Can you work these out from the model? Positions are in its coordinate system, mm. A direction names the side the tool comes from. Coordinates: 2 decimals unless noted, no trailing zeros. Order: outer loops, then holes, each group sorted by start corner. A loop starts at its lowest first (then second) coordinate and runs counter-clockwise, first axis right, second up.
```python
from build123d import *

# Parameters (mm, degrees)
F0_R     = 0.75
F0_R_2   = 1.5
F0_R_3   = 7.5
F1_DEPTH = 10
F2_T     = -2


with BuildPart() as f1:
    # F0 (on Front) → F1 (new body, symmetric)
    with BuildSketch(Plane.XZ):
        Polygon((37.5, 29), (37.5, 30), (-36.5, 30), (-37.5, 30), (-37.5, -29), (-37.5, -29.021632), (-37.5, -30), (37.488481, -30), (37.5, -30), align=None)
        with Locations((-35.74789, -28.249304)):
            Circle(F0_R, mode=Mode.SUBTRACT)
        with Locations((35.728708, -28.240002)):
            Circle(F0_R, mode=Mode.SUBTRACT)
        with Locations((-14, 0)):
            Circle(F0_R_2, mode=Mode.SUBTRACT)
        with Locations((-35.742357, 28.246674)):
            Circle(F0_R, mode=Mode.SUBTRACT)
        Circle(F0_R_3, mode=Mode.SUBTRACT)
        with Locations((14, 0)):
            Circle(F0_R_2, mode=Mode.SUBTRACT)
        with Locations((35.729614, 28.241964)):
            Circle(F0_R, mode=Mode.SUBTRACT)
    extrude(amount=F1_DEPTH, both=True)

    # F2
    f2_openings = [f1.faces().sort_by_distance(p)[0] for p in [
        (0, 10, 29.039531),
    ]]
    offset(amount=F2_T, openings=f2_openings)


solid = f1.part
```
1. Imagine slicing it at D-D on z = 23. Please give me the cut outline in (x, y), then the cut area to 3 significant figures.
Completed:
outline: (-37.5, -10) - (37.5, -10) - (37.5, 10) - (35.5, 10) - (35.5, -8) - (-35.5, -8) - (-35.5, 10) - (-37.5, 10) - close
area: 222 mm2
2. On a 3-axis mill with a long thin cutter (end or side, diameter ignored), from which of +Z, -Z, +X, -X, +Y, -Y can I reach the whole of each face in a straight line? I mean faces 3 (the flat face through (35.5, 1, 0)), 4 (the cylindrical face through (-35.84, 0.14, 28.99)). Say none if no direction works.
Completed:
face 3: +Y
face 4: +Y, -Y
3. Imagine slicing it at A-A on x = 14. Please give me the cut outline in (y, z), then the cut area to 3 significant figures.
Completed:
outline: (-10, -30) - (10, -30) - (10, -28) - (-8, -28) - (-8, -3.5) - (10, -3.5) - (10, -1.5) - (-10, -1.5) - close; (-10, 1.5) - (10, 1.5) - (10, 3.5) - (-8, 3.5) - (-8, 28) - (10, 28) - (10, 30) - (-10, 30) - close
area: 258 mm2
4. Thinking about a two-plate mould opening in X: for faces 1 (the flat face through (0, 1, 28)), 2 (the flat face through (1, 10, 8)), which applies, pulls with the +X half, pulls with the -X half, needs draft (parallel to the pull), parting line crosses it, or undercut?
Completed:
face 1: undercut
face 2: needs draft
5. Imagine slicing it at B-B on y = 0. Give the number of separate pieces and of enclosed holes in the cut face, then the cut area to 3 significant figures.
Completed:
separate pieces: 4
enclosed holes: 8
area: 705 mm2
6. Please list where these lines run through material, in increasing order: probe 1 along Z at (x, y) = (0, 5.5); probe 2 along Z at (x, y) = (-23, -0.75); probe 3 along X at (y, z) = (-1.75, -21.5).
Completed:
probe 1: z = -30 to -28, -9.5 to -7.5, 7.5 to 9.5, 28 to 30
probe 2: z = -30 to -28, 28 to 30
probe 3: x = -37.5 to -35.5, 35.5 to 37.5
7. I'm going to push flat-ended pins straight in: pin 1 (0.9 mm diameter, centred on x = 35.73, z = -28.24, fed in from +Y); pin 2 (3 mm diameter, centred on x = -14.5, z = -23, fed in from +Y). Where does each tip first touch, or does it pass through?
Completed:
pin 1: passes through
pin 2: stops at y = -8
